CAD build for the part. Positions are in the model's coordinates, mm. A direction names the side the tool comes from. Round coordinates to 2 decimals unless told otherwise and drop trailing zeros. Write each loop counter-clockwise with the first axis right and the second up, starting at its lowest first coordinate (ties: lowest second). Pieces come first, ordered by that corner, then holes. Notation, with made-up numbers: (54, 65.5) - (88, 65.5) arc R11 ccw to (88, 81.5) - close; hole circle Ø8 at (-7, 11.5). An arc over 180 degrees is marked (long way). Put each result on its own line as item: value. Start each with the question number.
Item 1: Cut at C-C (y = 124). Give the cut face in (x, z), and give its area (3 significant figures).
Item 2: Cut at D-D (x = 11). Give the cut face in (y, z).
Item 3: Cut at B-B (y = 104). Give the cut face in (x, z), and give its area (3 significant figures).
Item 4: 3-axis set-ups, long thin cutter, end or side, ignore diameter. For faces 1 (the cylindrical face through (52.59, 107.82, 70.67)), 2 (the flat face through (0, 93, 56)), 3 (the flat face through (53, 110, 67.5)): which of +Z, -Z, +X, -X, +Y, -Y reach the whole face in a straight line?
Item 5: Cut at A-A (z = 52). Give the cut face in (x, y), and give its area (3 significant figures).
Item 6: Mould opens along Y. For faces 4 (the flat face through (52, 0, 56)), 5 (the flat face through (52, 185, 55)), 6 (the flat face through (2, 173, 38)), 7 (the flat face through (52, 3, 55)) say: released by +Y, released by -Y, zero draft, split by the parting line, or undercut.
Item 7: Pin check, flat tips, straight feed: pin 1 Ø3 at (x, y) = (40, 110) entering from -Z; pin 2 Ø2.5 at (x, y) = (103, 45.5) entering from -Z; pin 3 Ø3.5 at (x, z) = (4, 38) entering from -Y. Stop position of each tip, or through.
Item 8: Drill centre lines: line 1 (X direction, y = 34.5, z = 70); line 2 (Y direction, x = 23.5, z = 63); line 3 (Y direction, x = 52, z = 68). Where is each one in solid material? Low to high. Write a range as from..to.
```python
from build123d import *

# Parameters (mm, degrees)
SKETCH016_W         = 106
SKETCH016_H         = 188
SKETCH016_W_2       = 96
SKETCH016_H_2       = 182
PAD010_DEPTH        = 31
SKETCH017_W         = 3
SKETCH017_H         = 15
SKETCH017_H_2       = 25
PAD011_DEPTH        = 3.8
SKETCH018_W         = 3.2
SKETCH018_H         = 15
POCKET006_DEPTH     = 17.5
SKETCH019_W         = 106
SKETCH019_H         = 188
SKETCH019_W_2       = 59
SKETCH019_H_2       = 10
PAD012_DEPTH        = 2
CHAMFER001_SIZE     = 0.8
CHAMFER002_SIZE     = 1.2
PAD013_DEPTH        = 2
LINEARPATTERN_COUNT = 30
LINEARPATTERN_PITCH = 1.896552
PAD014_DEPTH        = 59
FILLET_R            = 1.5


with BuildPart() as part:
    # Sketch016 → Pad010 (new body)
    with BuildSketch(Plane.XY):
        with Locations((53, 94)):
            Rectangle(SKETCH016_W, SKETCH016_H)
        with Locations((53, 94)):
            Rectangle(SKETCH016_W_2, SKETCH016_H_2, mode=Mode.SUBTRACT)
    extrude(amount=PAD010_DEPTH)

    # Sketch017 (on Face9 of Pad010) → Pad011 (join)
    with BuildSketch(Plane(origin=(0, 0, 0), x_dir=(1, 0, 0), z_dir=(0, 0, -1))):
        with Locations((3.5, -10.5)):
            Rectangle(SKETCH017_W, SKETCH017_H)
        with Locations((3.5, -172.5)):
            Rectangle(SKETCH017_W, SKETCH017_H_2)
        with Locations((102.5, -172.5)):
            Rectangle(SKETCH017_W, SKETCH017_H_2)
        with Locations((102.5, -10.5)):
            Rectangle(SKETCH017_W, SKETCH017_H)
    extrude(amount=PAD011_DEPTH)

    # Sketch018 (on Face4 of Pad011) → Pocket006 (cut)
    with BuildSketch(Plane(origin=(0, 0, 0), x_dir=(1, 0, 0), z_dir=(0, 0, -1))):
        with Locations((3.4, -48.5)):
            Rectangle(SKETCH018_W, SKETCH018_H)
        with Locations((102.6, -48.5)):
            Rectangle(SKETCH018_W, SKETCH018_H)
    extrude(amount=-POCKET006_DEPTH, mode=Mode.SUBTRACT)

    # Sketch019 (on Face5 of Pocket006) → Pad012 (join)
    with BuildSketch(Plane.XY.offset(31)):
        with Locations((53, 94)):
            Rectangle(SKETCH019_W, SKETCH019_H)
        with Locations((53, 105)):
            Rectangle(SKETCH019_W_2, SKETCH019_H_2, mode=Mode.SUBTRACT)
    extrude(amount=PAD012_DEPTH)

    # Chamfer001
    chamfer001_edges = [part.edges().sort_by_distance(p)[0] for p in [
        (101, 10.5, -3.8),
        (102.5, 18, -3.8),
        (104, 10.5, -3.8),
        (102.5, 3, -3.8),
        (102.5, 185, -3.8),
        (104, 172.5, -3.8),
        (102.5, 160, -3.8),
        (101, 172.5, -3.8),
        (5, 172.5, -3.8),
        (3.5, 3, -3.8),
        (2, 10.5, -3.8),
        (3.5, 18, -3.8),
        (5, 10.5, -3.8),
    ]]
    chamfer(chamfer001_edges, length=CHAMFER001_SIZE)

    # Chamfer002
    chamfer002_edges = [part.edges().sort_by_distance(p)[0] for p in [
        (102.6, 56, 0),
        (102.6, 41, 0),
        (3.4, 41, 0),
        (3.4, 56, 0),
    ]]
    chamfer(chamfer002_edges, length=CHAMFER002_SIZE)

    # Sketch020 (on Face12 of Chamfer002) → Pad013 (join)
    with BuildSketch(Plane(origin=(0, 0, 31), x_dir=(1, 0, 0), z_dir=(0, 0, -1))):
        Polygon((81.5, -100), (80.5, -102), (79.5, -100), align=None)
    pad013 = extrude(amount=-PAD013_DEPTH)

    # LinearPattern: Pad013 ×30
    with Locations(*[(-i * LINEARPATTERN_PITCH, 0, 0) for i in range(1, LINEARPATTERN_COUNT)]):
        add(pad013)

    # Sketch021 (on Face112 of LinearPattern) → Pad014 (join)
    with BuildSketch(Plane.YZ.offset(23.5)):
        with BuildLine():
            ThreePointArc((110, 33), (107.798766, 30.632491), (107, 27.5))
            Line((107, 27.5), (115, 27.5))
            Line((115, 27.5), (115, 31))
            Line((110, 31), (115, 31))
            Line((110, 33), (110, 31))
        make_face()
    extrude(amount=PAD014_DEPTH)

    # Fillet
    fillet_edges = [part.edges().sort_by_distance(p)[0] for p in [
        (53, 115, 31),
        (53, 115, 27.5),
    ]]
    fillet(fillet_edges, radius=FILLET_R)


with BuildPart() as part_1:
    # Body003 placement: moved
    add(part.part.moved(Location((0, 0, 40))))


solid = part_1.part
```
Output values:
1. outline: (0, 40) - (5, 40) - (5, 71) - (101, 71) - (101, 40) - (106, 40) - (106, 73) - (0, 73) - close
1. area: 522 mm2
2. outline: (0, 40) - (3, 40) - (3, 71) - (185, 71) - (185, 40) - (188, 40) - (188, 73) - (0, 73) - close
3. outline: (0, 40) - (5, 40) - (5, 71) - (23.5, 71) - (23.5, 73) - (0, 73) - close; (82.5, 71) - (101, 71) - (101, 40) - (106, 40) - (106, 73) - (82.5, 73) - close
3. area: 404 mm2
4. face 1: +Z
4. face 2: +Z, -Z, -X, +Y, -Y
4. face 3: -Z
5. outline: (0, 0) - (106, 0) - (106, 188) - (0, 188) - close; hole (1.8, 41) - (5, 41) - (5, 3) - (101, 3) - (101, 41) - (104.2, 41) - (104.2, 56) - (101, 56) - (101, 185) - (5, 185) - (5, 56) - (1.8, 56) - close
5. area: 2,360 mm2
6. face 4: released by -Y
6. face 5: undercut
6. face 6: zero draft
6. face 7: undercut
7. pin 1: z = 67.5
7. pin 2: z = 40
7. pin 3: y = 3
8. line 1: 0..5, 101..106
8. line 2: 0..3, 185..188
8. line 3: 0..3, 107.02..114.62, 185..188
